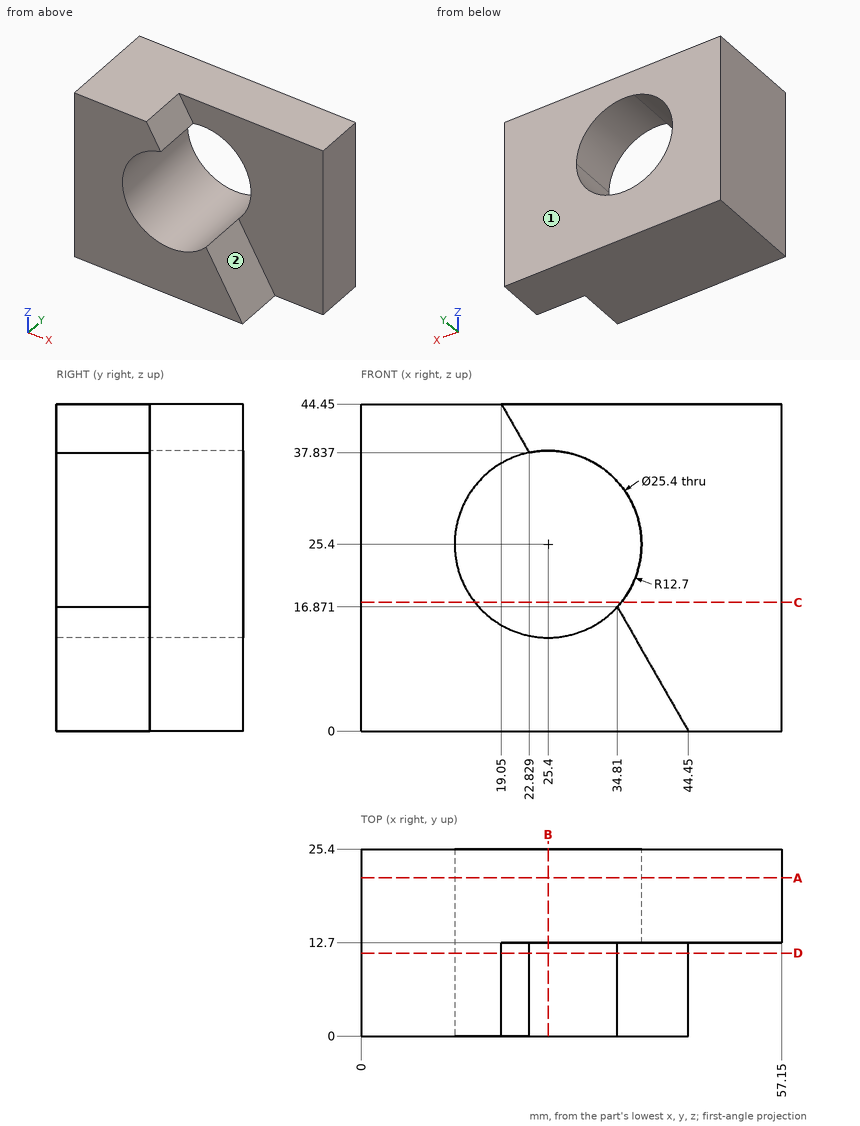
Input: dimensioned drawing with shaded views. Units: mm. Origin: part minimum x, y, z. A direction names the side the tool comes from. Round coordinates to 2 decimals unless told otherwise and drop trailing zeros. Loops run counter-clockwise (first coordinate to the right, second up) from the corner with the lowest first, then second, coordinate; pieces in that order, holes last.
1) Pin query (flat end, axial travel): pin 1 (1 mm diameter, centred on x = 38.5, y = 12, fed in from +Z); pin 2 (4 mm diameter, centred on y = 9, z = 33, fed in from +X) (1 decimal); pin 3 (8 mm diameter, centred on y = 9, z = 36.5, fed in from -X); pin 4 (11.5 mm diameter, centred on x = 40.5, z = 19.5, fed in from -Y). Return the tip coordinate at first contact, or that it passes through.
Ans:
pin 1: stops at z = 11.29
pin 2: stops at x = 17.1
pin 3: stops at x = 0
pin 4: stops at y = 12.7
2) Section query D-D on y = 11.25. Return the cut outline in (x, z).
Ans:
outline: (0, 0) - (44.45, 0) - (34.81, 16.87) arc R12.7 cw (long way) to (22.83, 37.84) - (19.05, 44.45) - (0, 44.45) - close
3) Section query A-A on y = 21.5. Return the cut outline in (x, z).
Ans:
outline: (0, 0) - (57.15, 0) - (57.15, 44.45) - (0, 44.45) - close; hole circle Ø25.4 at (25.4, 25.4)
4) Section query B-B on x = 25.4. Return the cut outline in (y, z).
Ans:
outline: (0, 0) - (25.4, 0) - (25.4, 12.7) - (0, 12.7) - close; (12.7, 38.1) - (25.4, 38.1) - (25.4, 44.45) - (12.7, 44.45) - close
5) Set-up query: the marked faces 1 and 2. Return all of +Z, -Z, +X, -X, +Y, -Y with unobstructed straight access to the full face (end or side cutting, diameter ignored); none if empty.
Ans:
face 1: +Z, -Z, +X, -X, +Y
face 2: +Z, +X, -Y
6) Section query C-C on z = 17.5. Return the cut outline in (x, y).
Ans:
outline: (0, 0) - (15.46, 0) - (15.46, 25.4) - (0, 25.4) - close; (35.34, 12.7) - (57.15, 12.7) - (57.15, 25.4) - (35.34, 25.4) - close
7) Material intervals for line 1 (Z direction, x = 25.4, y = 18.75); line 2 (X direction, y = 17.75, z = 25.4); line 3 (Z direction, x = 25.4, y = 8.75), sorted ascending.
Ans:
line 1: z = 0 to 12.7, 38.1 to 44.45
line 2: x = 0 to 12.7, 38.1 to 57.15
line 3: z = 0 to 12.7
